For this review, take the finished solid that the model builds, in its own axes (mm). A direction names the side the tool comes from. Round coordinates to 2 decimals unless told otherwise and drop trailing zeros. Loops run counter-clockwise (first coordinate to the right, second up) from the corner with the lowest first, then second, coordinate; pieces in that order, holes last.
1) Insertion check: pin 1 (12 mm diameter, centred on x = 56.5, y = 27, fed in from +Z). The pin has a flat end and moves straight along its axis. Give the tip position at first contact, or say it passes through.
2) Wall thickness on L1, parallel to Y at x = 4, z = 9.25; L2, parallel to X at y = -29, z = 11.5; L3, parallel to Z at x = -18, y = 71.5: over which ranges is each line inside the solid? List them lowest first.
3) Take a section at A-A (y = 78). State the section outline as (x, z) points.
4) Take a section at B-B (z = 8.5). State the section outline as (x, y) points.
5) Take a section at C-C (x = 8.5). State the section outline as (y, z) points, then the cut area to 3 significant figures.
6) Tool access review of faces 1 (the flat face through (-30, 6, 12.7)), 2 (the flat face through (-26.92, 7, 9)): name each direction out of +Z, -Z, +X, -X, +Y, -Y from which nothing blocks a thin tool from reaching the whole face with its end or side.
Autodesk Inventor part; units mm, degrees
ref_plane "YZ Plane" through (0, 0, 0) normal (1, 0, 0) x (0, 1, 0)
ref_plane "XZ Plane" through (0, 0, 0) normal (0, 1, 0) x (-1, 0, 0)
ref_plane "XY Plane" through (0, 0, 0) normal (0, 0, 1) x (1, 0, 0)
sketch "Sketch1" plane through (0, 0, 0) normal (0, 0, 1) x (1, 0, 0)
  line L0 (-31.9998, 94.2737) -> (95.0002, 94.2737)
  line L1 (95.0002, 94.2737) -> (95.0002, -83.5263)
  line L2 (95.0002, -83.5263) -> (-31.9998, -83.5263)
  line L3 (-31.9998, -83.5263) -> (-31.9998, 94.2737)
  point P0 (0, 0)
  dimension "d0" = 127
  dimension "d1" = 177.8
ref_plane "Work Plane1" through (0, 0, 6.35) normal (0, 0, 1) x (1, 0, 0)
sketch "Sketch3" plane through (0, 0, 6.35) normal (0, 0, 1) x (1, 0, 0)
  circle A0 centre (-6.5998, 81.5737) radius 1.7145
  line L0 (-57.3998, 94.2737) -> (-57.3998, -108.9263)
  circle A1 centre (69.6002, 81.5737) radius 1.7145
  circle A2 centre (-6.5998, -11.1363) radius 1.7145
  circle A3 centre (69.6002, -11.1363) radius 1.7145
  line L1 (95.0002, -108.9263) -> (95.0002, 94.2737)
  line L2 (95.0002, 94.2737) -> (-57.3998, 94.2737)
  point P0 (0, 0)
  dimension "d4" = 3.429
  dimension "d7" = 50.8
  dimension "d14" = 3.429
  dimension "d15" = 3.429
  dimension "d16" = 3.429
  dimension "d17" = 76.2
  dimension "d18" = 92.71
  dimension "d19" = 92.71
  dimension "d20" = 76.2
  dimension "d21" = 25.4
  dimension "d22" = 12.7
  dimension "d23" = 12.7
extrude "Extrusion3" add sketch "Sketch1" along normal blind 6.35
extrude "Extrusion4" cut sketch "Sketch3" against normal blind 6.35
sketch "Sketch4" plane through (0, 0, 6.35) normal (0, 0, 1) x (1, 0, 0)
  point P0 (0, 0)
sketch "Sketch6" plane through (0, 0, 6.35) normal (0, 0, 1) x (1, 0, 0)
  line L0 (-31.9998, 94.2737) -> (-31.9998, -83.5263)
  line L1 (-31.9998, 94.2737) -> (-26.9198, 94.2737)
  line L2 (-26.9198, 94.2737) -> (-26.9198, -83.5263)
  line L3 (-26.9198, -83.5263) -> (-31.9998, -83.5263)
  line L4 (-31.9998, -83.5263) -> (-31.9998, 94.2737)
  line L5 (95.0002, -83.5263) -> (95.0002, 94.2737)
  line L6 (-31.9998, -83.5263) -> (95.0002, -83.5263)
  line L7 (95.0002, 94.2737) -> (89.9202, 94.2737)
  line L8 (89.9202, 94.2737) -> (89.9202, -83.5263)
  line L9 (89.9202, -83.5263) -> (95.0002, -83.5263)
  line L10 (95.0002, -83.5263) -> (95.0002, 94.2737)
  line L11 (-26.9198, 94.2737) -> (89.9202, 94.2737)
  line L12 (89.9202, 94.2737) -> (89.9202, 89.1937)
  line L13 (89.9202, 89.1937) -> (-26.9198, 89.1937)
  line L14 (-26.9198, 89.1937) -> (-26.9198, 94.2737)
  line L15 (-26.9198, -83.5263) -> (89.9202, -83.5263)
  line L16 (89.9202, -83.5263) -> (89.9202, -78.4463)
  line L17 (89.9202, -78.4463) -> (-26.9198, -78.4463)
  line L18 (-26.9198, -78.4463) -> (-26.9198, -83.5263)
  point P0 (0, 0)
  dimension "d34" = 5.08
  dimension "d35" = 5.08
  dimension "d36" = 5.08
  dimension "d37" = 5.08
extrude "Extrusion5" add sketch "Sketch6" along normal blind 6.35 contours L1 L2 L3 L0
sketch "Sketch7" plane through (0, 0, 6.35) normal (0, 0, 1) x (1, 0, 0)
  line L0 (-26.9198, 94.2737) -> (-31.9998, 94.2737)
  line L1 (95.0002, -83.5263) -> (95.0002, 94.2737)
  line L2 (-26.9198, 94.2737) -> (95.0002, 94.2737)
  line L3 (95.0002, 94.2737) -> (95.0002, 89.1937)
  line L4 (95.0002, 89.1937) -> (-26.9198, 89.1937)
  line L5 (-26.9198, 89.1937) -> (-26.9198, 94.2737)
  point P0 (0, 0)
  dimension "d40" = 5.08
extrude "Extrusion6" add sketch "Sketch7" along normal blind 6.35
sketch "Sketch8" plane through (0, 0, 6.35) normal (0, 0, 1) x (1, 0, 0)
  line L0 (95.0002, 89.1937) -> (95.0002, 94.2737)
  line L1 (95.0002, 89.1937) -> (89.9202, 89.1937)
  line L2 (89.9202, 89.1937) -> (89.9202, -83.5263)
  line L3 (89.9202, -83.5263) -> (95.0002, -83.5263)
  line L4 (95.0002, -83.5263) -> (95.0002, 89.1937)
  point P0 (0, 0)
  dimension "d43" = 5.08
  dimension "d44" = 172.72
extrude "Extrusion7" add sketch "Sketch8" along normal blind 6.35
sketch "Sketch9" plane through (0, 0, 6.35) normal (0, 0, 1) x (1, 0, 0)
  line L0 (89.9202, 89.1937) -> (89.9202, -83.5263)
  line L1 (89.9202, -83.5263) -> (-26.9198, -83.5263)
  line L2 (-26.9198, -83.5263) -> (-26.9198, -78.4463)
  line L3 (-26.9198, -78.4463) -> (89.9202, -78.4463)
  line L4 (89.9202, -78.4463) -> (89.9202, -83.5263)
  point P0 (0, 0)
  dimension "d47" = 116.84
  dimension "d48" = 5.08
extrude "Extrusion8" add sketch "Sketch9" along normal blind 6.35
properties part number "Robot_Base"
Response:
1. pin 1: stops at z = 6.35
2. L1: y = -83.53 to -78.45, 89.19 to 94.27
2. L2: x = -32 to -26.92, 89.92 to 95
2. L3: z = 0 to 6.35
3. outline: (-32, 0) - (95, 0) - (95, 12.7) - (89.92, 12.7) - (89.92, 6.35) - (-26.92, 6.35) - (-26.92, 12.7) - (-32, 12.7) - close
4. outline: (-32, -83.53) - (95, -83.53) - (95, 94.27) - (-32, 94.27) - close; hole (-26.92, -78.45) - (89.92, -78.45) - (89.92, 89.19) - (-26.92, 89.19) - close
5. outline: (-83.53, 0) - (94.27, 0) - (94.27, 12.7) - (89.19, 12.7) - (89.19, 6.35) - (-78.45, 6.35) - (-78.45, 12.7) - (-83.53, 12.7) - close
5. area: 1,190 mm2
6. face 1: +Z, +X, -X, +Y, -Y
6. face 2: +Z
